from build123d import *

# Parameters (mm, degrees)
F1_DEPTH = 3.175
F2_R     = 1.27
F3_DEPTH = 1.524
F4_R     = 1.27


with BuildPart() as f1:
    # F0 (on Front) → F1 (new body, symmetric)
    with BuildSketch(Plane.XZ):
        Polygon((-14.605, -4.064), (-6.35, -4.064), (-6.35, 0), (6.35, 0), (6.35, -4.064), (14.605, -4.064), (14.605, -2.54), (7.874, -2.54), (7.874, 1.524), (-7.874, 1.524), (-7.874, -2.54), (-14.605, -2.54), align=None)
    extrude(amount=F1_DEPTH, both=True)

    # F2 (on face) → F3 (cut, through all)
    with BuildSketch(Plane.XY.offset(-2.54)):
        with Locations((-11.2395, 0)):
            Circle(F2_R)
        with Locations((11.2395, 0)):
            Circle(F2_R)
    extrude(amount=-F3_DEPTH, mode=Mode.SUBTRACT)

    # F4
    f4_edges = [f1.edges().sort_by_distance(p)[0] for p in [
        (-6.35, 0, 0),
        (6.35, 0, 0),
        (-7.874, 0, -2.54),
        (7.874, 0, -2.54),
    ]]
    fillet(f4_edges, radius=F4_R)


solid = f1.part
Could you check a few things on this model? Use its own coordinates, in mm. A direction names the side the tool comes from. Round coordinates to 2 decimals unless told otherwise and drop trailing zeros. Write each loop counter-clockwise with the first axis right and the second up, starting at its lowest first coordinate (ties: lowest second). Pieces come first, ordered by that corner, then holes. Notation, with made-up numbers: (8.5, 72) - (33.5, 72) arc R15 cw to (33.5, 79) - close; hole circle Ø10 at (31, 60.5). An arc over 180 degrees is marked (long way). Use a Markdown table: item, result.
Q1. Thinking about a two-plate mould opening in X: for faces 6 (the flat face through (0, 0, 1.524)), 7 (the cylindrical face through (12.41, -0.49, -3.29)), 8 (the cylindrical face through (-11.4, 1.26, -3.29)), 9 (the flat face through (-7.874, 0, 0)), which applies, released by +X, released by -X, zero draft, split by the parting line, or undercut?
Output values:
| item | result |
|---|---|
| face 6 | zero draft |
| face 7 | undercut |
| face 8 | undercut |
| face 9 | released by -X |
Q2. Please list where these lines run through material, in increasing order: L1, parallel to X at y = -1, z = 0.45; L2, parallel to Z at x = -0.5, y = 1.5; L3, parallel to X at y = 2.5, z = -3.3 (3 decimals).
Output values:
| item | result |
|---|---|
| L1 | -7.87 to 7.87 |
| L2 | 0 to 1.52 |
| L3 | -14.605 to -6.35, 6.35 to 14.605 |
Q3. For faces 1 (the flat face through (13, 0, -2.54)), 2 (the flat face through (-13, 0, -2.54)), 3 (the flat face through (-9.6, 0, -4.064)), 4 (the flat face through (-14.605, 0, -3)), 5 (the flat face through (0, 0, 0)), which set-ups out of +Z, -Z, +X, -X, +Y, -Y let a thin tool reach every point of the face, with its end or its side?
Output values:
| item | result |
|---|---|
| face 1 | +Z, +X, +Y, -Y |
| face 2 | +Z, -X, +Y, -Y |
| face 3 | -Z, +X, -X, +Y, -Y |
| face 4 | +Z, -Z, -X, +Y, -Y |
| face 5 | -Z, +Y, -Y |
Q4. I want a section at A-A (z = -2.85). Count the separate pieces of the cut face and the enclosed holes in it, plus the area to 3 significant figures.
Output values:
| item | result |
|---|---|
| separate pieces | 2 |
| enclosed holes | 2 |
| area | 94.7 mm2 |
Q5. For pin 1 (0.8 mm diameter, centred on y = 0, z = 0.5, fed in from -X); pin 2 (1.4 mm diameter, centred on y = -1.5, z = 0, fed in from +X); pin 3 (2 mm diameter, centred on x = 11.24, y = 0, fed in from +Z), each with a flat end and sliding along its axis, tell me the tip position at first contact or that it passes through.
Output values:
| item | result |
|---|---|
| pin 1 | x = -7.87 |
| pin 2 | x = 7.87 |
| pin 3 | through |
Q6. I want a section at C-C (x = -12). List the corners of the cut face in (y, z) for me (3 decimals).
Output values:
| item | result |
|---|---|
| outline | (-3.175, -4.064) - (-1.017, -4.064) - (-1.017, -2.54) - (-3.175, -2.54) - close; (1.017, -4.064) - (3.175, -4.064) - (3.175, -2.54) - (1.017, -2.54) - close |
Q7. I want a section at D-D (z = -1.6). List the corners of the cut face in (x, y) for me (3 decimals), plus the area to 3 significant figures.
Output values:
| item | result |
|---|---|
| outline | (-7.918, -3.175) - (-6.35, -3.175) - (-6.35, 3.175) - (-7.918, 3.175) - close; (6.35, -3.175) - (7.918, -3.175) - (7.918, 3.175) - (6.35, 3.175) - close |
| area | 19.9 mm2 |
